Input: part model. Units: mm. Frame: model coordinates. Face numbers are marked on the shaded views. A direction names the side the tool comes from. Coordinates: 2 decimals unless noted, no trailing zeros. Loops run counter-clockwise (first coordinate to the right, second up) from the corner with the lowest first, then second, coordinate; pieces in that order, holes last. Notation, with made-up numbers: (-5, 11.25) - (40, 11.25) arc R24 cw to (40, 34.25) - close; hole circle Ø8 at (45.25, 21.25). An arc over 180 degrees is marked (long way). Answer as CSV lines item,"result". Start each with the question number.
```python
from build123d import *

# Parameters (mm, degrees)
HOLE_WIZARD_M3_1_D       = 2.5
PATTERN_CIRCULAR_1_COUNT = 4
SKETCH_5_R               = 2.25
EXTRUDE_1_DEPTH          = 9
HOLE_WIZARD_M3_2_D       = 2.5
HOLE_WIZARD_M3_2_DEPTH   = 12
HOLE_WIZARD_M3_2_TIP     = 0.751075774


with BuildPart() as part:
    # Model → 旋转1 (revolve)
    with BuildSketch(Plane.XY, mode=Mode.PRIVATE) as revolve_1_sk:
        Polygon((0, 32), (0, 0), (2.5, 0), (2.5, 4), (3, 4), (3, 9.6), (4, 9.6), (4, 11.6), (10, 11.6), (10, 20.4), (4, 20.4), (4, 22.4), (3, 22.4), (3, 28), (2.5, 28), (2.5, 32), align=None)
    revolve(revolve_1_sk.sketch.rotate(Axis((0, 32, 0), (0, -1, 0)), 180), axis=Axis((0, 32, 0), (0, -1, 0)))

    # M3 螺纹孔1 (through all)
    with Locations(Plane(origin=(0, 11.6, 7), x_dir=(-1, 0, 0), z_dir=(0, -1, 0))):
        with Locations((0, 0)):
            hole_wizard_m3_1 = Hole(HOLE_WIZARD_M3_1_D / 2)

    # 阵列(圆周)1: M3 螺纹孔1 ×4 about axis
    pattern_circular_1_axis = Axis((0, 0, 0), (0, 1, 0))
    for i in range(1, PATTERN_CIRCULAR_1_COUNT):
        add(hole_wizard_m3_1.rotate(pattern_circular_1_axis, i * 360 / PATTERN_CIRCULAR_1_COUNT), mode=Mode.SUBTRACT)

    # 草图5 → 凸台-拉伸1 (add)
    with BuildSketch(Plane.XZ):
        Circle(SKETCH_5_R)
    extrude(amount=EXTRUDE_1_DEPTH)

    # M3 螺纹孔2
    with Locations(Plane(origin=(0, -9, 0), x_dir=(-1, 0, 0), z_dir=(0, -1, 0))):
        with Locations((0, 0)):
            Hole(HOLE_WIZARD_M3_2_D / 2, depth=HOLE_WIZARD_M3_2_DEPTH)
            with Locations((0, 0, -(HOLE_WIZARD_M3_2_DEPTH + HOLE_WIZARD_M3_2_TIP / 2))):  # 118° drill point
                Cone(0, HOLE_WIZARD_M3_2_D / 2, HOLE_WIZARD_M3_2_TIP, mode=Mode.SUBTRACT)


solid = part.part
```
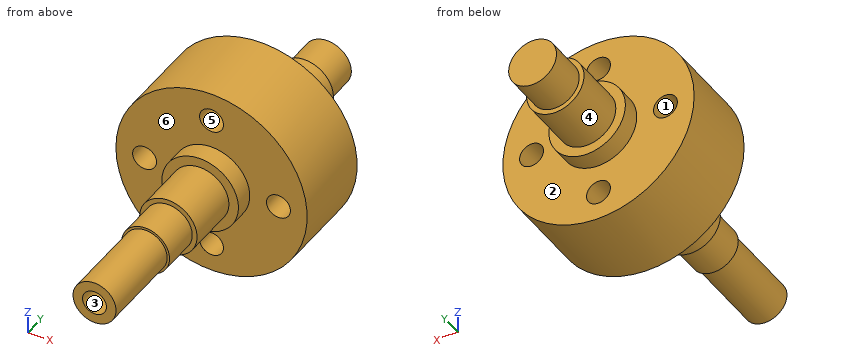
Item 1: Draft query along Z for the marked faces 4, 5 and 6. Return one class per face: pulls with the +Z half, pulls with the -Z half, needs draft (parallel to the pull), parting line crosses it, or undercut.
Item 2: Section query D-D, the plane y = 14.5. Output: boundary loops of the cut face in (x, z), and give its area (3 significant figures).
Item 3: Section query A-A, the plane x = -6.5. Output: boundary loops of the cut face in (y, z).
Item 4: Set-up query: the marked faces 1, 2 and 3. Return all of +Z, -Z, +X, -X, +Y, -Y with unobstructed straight access to the full face (end or side cutting, diameter ignored); none if empty.
Item 5: Section query B-B, the plane z = -7. Output: boundary loops of the cut face in (x, y), and give its area (3 significant figures).
Item 6: Material intervals for probe 1 along Z at (x, y) = (0, 17.75); probe 2 along Y at (x, z) = (-2.25, -4.5); probe 3 along Y at (x, z) = (1, 3.25), sorted ascending.
Item 7: Contact query for flat-ended pins moving along their axis: P1, Ø6, axis at x = -3, z = -5, coming from the +Y side; P2, Ø3, axis at x = -7, z = 0, coming from the -Y side; P3, Ø2, axis at x = 2, y = 25, coming from the -Z side. Output: stop coordinate, or through.
Item 8: Section query C-C, the plane y = 1.5. Output: boundary loops of the cut face in (x, z), and give its area (3 significant figures).
Response values:
1,face 4,"parting line crosses it"
1,face 5,"undercut"
1,face 6,"needs draft"
2,outline,"circle Ø20 at (0, 0); hole circle Ø2.5 at (-7, 0); hole circle Ø2.5 at (0, -7); hole circle Ø2.5 at (0, 7); hole circle Ø2.5 at (7, 0)"
2,area,"295 mm²"
3,outline,"(11.6, -7.6) - (20.4, -7.6) - (20.4, -1.15) - (11.6, -1.15) - close; (11.6, 1.15) - (20.4, 1.15) - (20.4, 7.6) - (11.6, 7.6) - close"
4,face 1,"+Y, -Y"
4,face 2,"+Y"
4,face 3,"-Y"
5,outline,"(-7.14, 11.6) - (-1.25, 11.6) - (-1.25, 20.4) - (-7.14, 20.4) - close; (1.25, 11.6) - (7.14, 11.6) - (7.14, 20.4) - (1.25, 20.4) - close"
5,area,"104 mm²"
6,probe 1,"z = -10 to -8.25, -5.75 to 5.75, 8.25 to 10"
6,probe 2,"y = 11.6 to 20.4"
6,probe 3,"y = 9.6 to 22.4"
7,P1,"stops at y = 28"
7,P2,"stops at y = 11.6"
7,P3,"stops at z = -2.83"
8,outline,"circle Ø5 at (0, 0); hole circle Ø2.5 at (0, 0)"
8,area,"14.7 mm²"
